Verification items for the finished model (mm, model axes). Give positions to 0.01 mm unless a question says otherwise; leave off trailing zeros. Order: outer loops, then holes, each group sorted by start corner. A loop starts at its lowest first (then second) coordinate and runs counter-clockwise, first axis right, second up. Notation, with made-up numbers: (12.5, 20.25) -> (47.5, 20.25) arc R3 cw to (47.5, 25.25) -> close; hole circle Ø2 at (61, 1.25). An arc over 180 degrees is marked (long way). One line per question, with ' | ' between items. Start each with the question number.
Q1. Section check B-B on y = 8.5. Record the cut outline in (x, z), plus the area to 3 significant figures.
Q2. Material ranges on probe 1 along X at (y, z) = (6, -11); probe 2 along Z at (x, y) = (-10, 4); probe 3 along Z at (x, y) = (5, 5.25), recorded low to high. Write a range as [from, to].
Q3. Section check C-C on x = -5. Record the cut outline in (y, z), plus the area to 3 significant figures.
Q4. Section check A-A on z = 0. Record the cut outline in (x, y), plus the area to 3 significant figures.
Q5. Go/stop test with flat-tipped pins: pin 1 (3 mm diameter, centred on x = 5, z = 0, fed in from -Y); pin 2 (2 mm diameter, centred on x = -11, z = 11, fed in from +Y); pin 3 (3 mm diameter, centred on x = -15, y = 4, fed in from +Z); pin 4 (5 mm diameter, centred on x = 12, y = 3, fed in from +Z). Record where each tip stops, or that it passes through.
Q6. Section check D-D on z = -11. Record the cut outline in (x, y), plus the area to 3 significant figures.
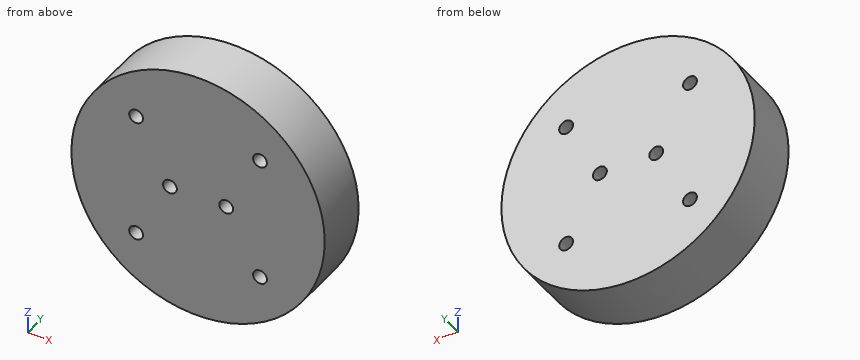
Autodesk Inventor part; units mm, degrees
ref_plane "YZ Plane" through (0, 0, 0) normal (1, 0, 0) x (0, 1, 0)
ref_plane "XZ Plane" through (0, 0, 0) normal (0, 1, 0) x (-1, 0, 0)
ref_plane "XY Plane" through (0, 0, 0) normal (0, 0, 1) x (1, 0, 0)
sketch "Эскиз1" plane through (0, 0, 0) normal (0, 1, 0) x (-1, 0, 0)
  circle A0 centre (0, 0) radius 22.5
  dimension "d0" = 45
extrude "Выдавливание1" add sketch "Эскиз1" along normal blind 10
sketch "Эскиз2" plane through (0, 10, 0) normal (0, 1, 0) x (1, 0, 0)
  line L0 (0, 0) -> (-5, 0)
  line L1 (-5, 0) -> (5, 0)
  dimension "d3" = 5
  dimension "d4" = 10
hole "Отверстие1" at (-5, 10, 0) at (5, 10, 0) direction (0, -1, 0) diameter 2.459 end through all
sketch "Эскиз3" plane through (0, 10, 0) normal (0, 1, 0) x (1, 0, 0)
  point P0 (0, 0)
sketch "Эскиз4" plane through (0, 0, 0) normal (0, -1, 0) x (1, 0, 0)
  line L0 (15.5563, 15.5563) -> (-15.5563, 15.5563)
  line L1 (-15.5563, 15.5563) -> (-15.5563, -15.5563)
  line L2 (-15.5563, -15.5563) -> (15.5563, -15.5563)
  line L3 (15.5563, -15.5563) -> (15.5563, 15.5563)
  line L4 (15.5563, 15.5563) -> (-15.5563, -15.5563)
  line L5 (15.5563, -15.5563) -> (-15.5563, 15.5563)
  line L6 (-11, 11) -> (11, 11)
  line L7 (11, 11) -> (11, -11)
  line L8 (11, -11) -> (-11, -11)
  line L9 (-11, -11) -> (-11, 11)
  point P0 (0, 0)
  dimension "d23" = 22
hole "Отверстие2" at (11, 0, -11) at (-11, 0, 11) at (11, 0, 11) at (-11, 0, -11) direction (0, 1, 0) diameter 2.459 end through all
properties part number "Диск (маховик, вал)"
Filled in:
1) outline: circle Ø45 at (0, 0); hole circle Ø2.46 at (-11, -11); hole circle Ø2.46 at (-11, 11); hole circle Ø2.46 at (-5, 0); hole circle Ø2.46 at (5, 0); hole circle Ø2.46 at (11, -11); hole circle Ø2.46 at (11, 11) | area: 1,560 mm²
2) probe 1: [-19.63, -12.23], [-9.77, 9.77], [12.23, 19.63] | probe 2: [-20.16, -11.72], [-10.28, 10.28], [11.72, 20.16] | probe 3: [-21.94, -1.23], [1.23, 21.94]
3) outline: (0, -21.94) -> (10, -21.94) -> (10, -1.23) -> (0, -1.23) -> close; (0, 1.23) -> (10, 1.23) -> (10, 21.94) -> (0, 21.94) -> close | area: 414 mm²
4) outline: (-22.5, 0) -> (-6.23, 0) -> (-6.23, 10) -> (-22.5, 10) -> close; (-3.77, 0) -> (3.77, 0) -> (3.77, 10) -> (-3.77, 10) -> close; (6.23, 0) -> (22.5, 0) -> (22.5, 10) -> (6.23, 10) -> close | area: 401 mm²
5) pin 1: y = 0 | pin 2: through | pin 3: z = 18 | pin 4: z = 20.4
6) outline: (-19.63, 0) -> (-12.23, 0) -> (-12.23, 10) -> (-19.63, 10) -> close; (-9.77, 0) -> (9.77, 0) -> (9.77, 10) -> (-9.77, 10) -> close; (12.23, 0) -> (19.63, 0) -> (19.63, 10) -> (12.23, 10) -> close | area: 343 mm²
